```python
from build123d import *

# Parameters (mm, degrees)
F0_W      = 33
F0_H      = 35
F0_W_2    = 8.5
F0_H_2    = 1.25
F1_DEPTH  = 1.5
F2_R      = 1
F3_DEPTH  = 1.5
F4_R      = 3
F5_R      = 10
F6_R      = 1
F7_DEPTH  = 1.5
F8_R      = 1.5
F8_R_2    = 1
F9_DEPTH  = 1
F10_R     = 1.5
F10_R_2   = 1
F11_DEPTH = 1
F12_R     = 1.5
F12_R_2   = 1
F13_DEPTH = 1


with BuildPart() as f1:
    # F0 (on Top) → F1 (new body)
    with BuildSketch(Plane.XY):
        with Locations((5.4070419595, 0)):
            Rectangle(F0_W, F0_H)
        with Locations((4.6570419595, 0)):
            Rectangle(F0_W_2, F0_H_2, mode=Mode.SUBTRACT)
    extrude(amount=-F1_DEPTH)

    # F2 (on face) → F3 (cut)
    with BuildSketch(Plane.XY):
        with Locations((-9.0911619139, 15.4008569585)):
            Circle(F2_R)
        with Locations((-9.0490024113, 7.7360985084)):
            Circle(F2_R)
        with Locations((-9.0064505073, 0)):
            Circle(F2_R)
        with Locations((-8.9662096661, -7.3159384689)):
            Circle(F2_R)
        with Locations((-8.9248921722, -14.8276165128)):
            Circle(F2_R)
    extrude(amount=-F3_DEPTH, mode=Mode.SUBTRACT)

    # F4
    f4_edges = [f1.edges().sort_by_distance(p)[0] for p in [
        (-11.092958, -17.5, -0.75),
        (-11.092958, 17.5, -0.75),
    ]]
    fillet(f4_edges, radius=F4_R)

    # F5
    f5_edges = [f1.edges().sort_by_distance(p)[0] for p in [
        (21.907042, 17.5, -0.75),
        (21.907042, -17.5, -0.75),
    ]]
    fillet(f5_edges, radius=F5_R)

    # F6 (on face) → F7 (join)
    with BuildSketch(Plane.XY):
        with Locations((11.9070419595, 0)):
            Circle(F6_R)
        with Locations((15.9070419595, 0)):
            Circle(F6_R)
        with Locations((19.9070419595, 0)):
            Circle(F6_R)
    extrude(amount=F7_DEPTH)

    # F8 (on face) → F9 (join)
    with BuildSketch(Plane.XY.offset(1.5)):
        with Locations((11.9070419595, 0)):
            Circle(F8_R)
        with Locations((11.9070419595, 0)):
            Circle(F8_R_2, mode=Mode.SUBTRACT)
        with Locations((11.9070419595, 0)):
            Circle(F8_R_2)
    extrude(amount=F9_DEPTH)

    # F10 (on face) → F11 (join)
    with BuildSketch(Plane.XY.offset(1.5)):
        with Locations((15.9070419595, 0)):
            Circle(F10_R)
        with Locations((15.9070419595, 0)):
            Circle(F10_R_2, mode=Mode.SUBTRACT)
        with Locations((15.9070419595, 0)):
            Circle(F10_R_2)
    extrude(amount=F11_DEPTH)

    # F12 (on face) → F13 (join)
    with BuildSketch(Plane.XY.offset(1.5)):
        with Locations((19.9070419595, 0)):
            Circle(F12_R)
        with Locations((19.9070419595, 0)):
            Circle(F12_R_2, mode=Mode.SUBTRACT)
        with Locations((19.9070419595, 0)):
            Circle(F12_R_2)
    extrude(amount=F13_DEPTH)


solid = f1.part
```
Check sheet for the modelled part. Datum: model origin and axes. Units: mm. A direction names the side the tool comes from. Give positions to 0.01 mm unless a question says otherwise; leave off trailing zeros. Loops run counter-clockwise (first coordinate to the right, second up) from the corner with the lowest first, then second, coordinate; pieces in that order, holes last. Notation, with made-up numbers: M -0.5,59.25 L 38.5,59.25 A19 cw 38.5,76.25 Z; hole C 46.5,8 d10. An arc over 180 degrees is marked long. Answer in a Markdown table with one row per item.
1) Cross-section at A-A (x = 4). Enter the section's corners in (y, z) (3 decimals).
Solutions:
| item | result |
|---|---|
| outline | M -17.5,-1.5 L -0.625,-1.5 L -0.625,0 L -17.5,0 Z; M 0.625,-1.5 L 17.5,-1.5 L 17.5,0 L 0.625,0 Z |
2) Thickness scan on line 1 (Z direction, x = 6, y = -10); line 2 (Y direction, x = 1, z = -0.7) (3 decimals); line 3 (X direction, y = 14, z = -0.3). Record the ranges inside material, lowest first.
Solutions:
| item | result |
|---|---|
| line 1 | z = -1.5 to 0 |
| line 2 | y = -17.5 to -0.625, 0.625 to 17.5 |
| line 3 | x = -11.09 to 19.51 |
3) Tool access check on faces 1 (the face through (2, -17.5, -1)), 2 (the face through (0.407, 0, -1)), 3 (the face through (13.293, -0.575, 1.993)). Record the directions out of +Z, -Z, +X, -X, +Y, -Y that give a thin tool (end or side, any length) a straight path to the whole face; none if there is none.
Solutions:
| item | result |
|---|---|
| face 1 | +Z, -Z, +X, -X, -Y |
| face 2 | +Z, -Z |
| face 3 | +Z |
4) Mould release check, pull along Y, two halves, no side actions. Record for faces 4 (the face through (20.83, -0.38, 0.74)), 5 (the face through (21.907, 0, -1)), 6 (the face through (-8.01, -7.02, -0.74)): released by +Y, released by -Y, zero draft, split by the parting line, or undercut.
Solutions:
| item | result |
|---|---|
| face 4 | split by the parting line |
| face 5 | zero draft |
| face 6 | undercut |
5) Depth check by flat-ended pin: pin 1 (1.2 mm diameter, centred on x = -8.92, y = -14.83, fed in from -Z); pin 2 (3 mm diameter, centred on x = -8.97, y = -7.32, fed in from +Z); pin 3 (2.5 mm diameter, centred on x = -9.05, y = 7.74, fed in from -Z). Enter the tip coordinate at first touch or a pass-through.
Solutions:
| item | result |
|---|---|
| pin 1 | passes through |
| pin 2 | stops at z = 0 |
| pin 3 | stops at z = -1.5 |
6) Cross-section at C-C (z = -0.5). Enter the section's corners in (x, y) (3 decimals).
Solutions:
| item | result |
|---|---|
| outline | M -11.093,-14.5 A3 ccw -8.093,-17.5 L 11.907,-17.5 A10 ccw 21.907,-7.5 L 21.907,7.5 A10 ccw 11.907,17.5 L -8.093,17.5 A3 ccw -11.093,14.5 Z; hole C -9.091,15.401 d2; hole C -9.049,7.736 d2; hole C -9.006,0 d2; hole C -8.966,-7.316 d2; hole C -8.925,-14.828 d2; hole M 0.407,-0.625 L 8.907,-0.625 L 8.907,0.625 L 0.407,0.625 Z |
7) Cross-section at D-D (x = 20.5). Enter the section's corners in (y, z), plus the area to 3 significant figures.
Solutions:
| item | result |
|---|---|
| outline | M -12.61,-1.5 L 12.61,-1.5 L 12.61,0 L 0.81,0 L 0.81,1.5 L 1.38,1.5 L 1.38,2.5 L -1.38,2.5 L -1.38,1.5 L -0.81,1.5 L -0.81,0 L -12.61,0 Z |
| area | 43.0 mm^2 |
8) Cross-section at B-B (y = 0). Count the separate pieces of the cut face and the enclosed holes in it, plus the area to 4 significant figures.
Solutions:
| item | result |
|---|---|
| separate pieces | 3 |
| enclosed holes | 0 |
| area | 51.75 mm^2 |
